Can you work these out from the model? Positions are in its coordinate system, mm. A direction names the side the tool comes from. Give positions to 0.01 mm unless a question says otherwise; leave off trailing zeros. Order: outer loops, then holes, each group sorted by start corner. A loop starts at its lowest first (then second) coordinate and runs counter-clockwise, first axis right, second up. Notation, with made-up numbers: (-7, 40) - (28, 40) arc R12 cw to (28, 53) - close; hole circle Ø11 at (34, 13.5). An arc over 180 degrees is marked (long way). Return JSON: item names as keys, results as strings.
```python
from build123d import *

# Parameters (mm, degrees)
SKETCH1_W           = 21
SKETCH1_H           = 30
SKETCH1_R           = 1.6
BOSS_EXTRUDE3_DEPTH = 10
SKETCH3_W           = 8
SKETCH3_H           = 30
BOSS_EXTRUDE4_DEPTH = 55
SKETCH4_W           = 30
SKETCH4_H           = 10
BOSS_EXTRUDE5_DEPTH = 25
CUT_EXTRUDE1_REACH  = 82.312
SKETCH5_W           = 6.5
SKETCH5_H           = 16.5
SKETCH7_R           = 2.5
CUT_EXTRUDE2_DEPTH  = 17.2
FILLET2_R           = 5
BOSS_EXTRUDE7_START = -10
BOSS_EXTRUDE7_DEPTH = 10


with BuildPart() as part:
    # Sketch1 → Boss-Extrude3 (new body)
    with BuildSketch(Plane(origin=(0, 0, 0), x_dir=(1, 0, 0), z_dir=(0, 1, 0))):
        with Locations((-4.5, -10)):
            Rectangle(SKETCH1_W, SKETCH1_H)
        with Locations(Location((0, 0, 0), (0, 0, 270))):
            Circle(SKETCH1_R, mode=Mode.SUBTRACT)
        with Locations(Location((0, -20, 0), (0, 0, 270))):
            Circle(SKETCH1_R, mode=Mode.SUBTRACT)
    extrude(amount=BOSS_EXTRUDE3_DEPTH)

    # Sketch3 → Boss-Extrude4 (add)
    with BuildSketch(Plane(origin=(0, 10, 0), x_dir=(1, 0, 0), z_dir=(0, 1, 0))):
        with Locations((-11, -10)):
            Rectangle(SKETCH3_W, SKETCH3_H)
    extrude(amount=BOSS_EXTRUDE4_DEPTH)

    # Sketch4 → Boss-Extrude5 (add)
    with BuildSketch(Plane.ZY.offset(15)):
        with Locations((10, 60)):
            Rectangle(SKETCH4_W, SKETCH4_H)
    extrude(amount=BOSS_EXTRUDE5_DEPTH)

    # Sketch5 → Cut-Extrude1 (cut, up to next)
    with BuildSketch(Plane(origin=(0, 65, 0), x_dir=(1, 0, 0), z_dir=(0, 1, 0)), mode=Mode.PRIVATE) as cut_extrude1_sk1:
        with Locations((-31.75, -10)):
            Rectangle(SKETCH5_W, SKETCH5_H)
    cut_extrude1_tool1 = extrude(cut_extrude1_sk1.sketch, amount=-CUT_EXTRUDE1_REACH, mode=Mode.PRIVATE) & part.part
    add(cut_extrude1_tool1.solids().sort_by_distance((-31.75, 65, 10))[0], mode=Mode.SUBTRACT)

    # Sketch7 → Cut-Extrude2 (cut)
    with BuildSketch(Plane.ZY.offset(40)):
        with Locations((10, 60)):
            Circle(SKETCH7_R)
    extrude(amount=-CUT_EXTRUDE2_DEPTH, mode=Mode.SUBTRACT)

    # Fillet2
    fillet2_edges = [part.edges().sort_by_distance(p)[0] for p in [
        (-7, 65, 10),
        (-15, 55, 10),
        (-40, 60, -5),
        (-40, 60, 25),
        (-15, 0, 10),
        (6, 5, -5),
        (6, 5, 25),
    ]]
    fillet(fillet2_edges, radius=FILLET2_R)

    # Sketch8 → Boss-Extrude7 (add)
    with BuildSketch(Plane.XY.offset(25).offset(BOSS_EXTRUDE7_START)):
        Polygon((-7, 10), (-7, 60), (6, 10), align=None)
    extrude(amount=-BOSS_EXTRUDE7_DEPTH)


solid = part.part
```
1. Suppose I cut it at C-C (z = 10). List the corners of the cut face in (x, y) for me, plus the area to 3 significant figures.
Checks:
{"outline": "(-40, 55) - (-35, 55) - (-35, 57.5) - (-40, 57.5) - close; (-40, 62.5) - (-35, 62.5) - (-35, 65) - (-40, 65) - close; (-28.5, 55) - (-20, 55) arc R5 cw to (-15, 50) - (-15, 5) arc R5 ccw to (-10, 0) - (6, 0) - (6, 10) - (-7, 60) arc R5 ccw to (-12, 65) - (-28.5, 65) - (-28.5, 62.5) - (-22.8, 62.5) - (-22.8, 57.5) - (-28.5, 57.5) - close", "area": "1,100 mm^2"}
2. Suppose I cut it at B-B (x = -32.5). List the corners of the cut face in (y, z) for me.
Checks:
{"outline": "(55, -5) - (65, -5) - (65, 1.75) - (55, 1.75) - close; (55, 18.25) - (65, 18.25) - (65, 25) - (55, 25) - close"}
3. For pin 1 Ø3 at (y, z) = (60, 10) entering from +X; pin 2 Ø8 at (x, z) = (-0.5, 22) entering from +Y; pin 3 Ø6.5 at (x, y) = (0.5, 45.5) entering from -Z; pin 4 Ø3 at (y, z) = (24.5, 4) entering from -X, each with a flat end and sliding along its axis, tell me the tip position at first contact or that it passes through.
Checks:
{"pin 1": "x = -6.61", "pin 2": "y = 10", "pin 3": "through", "pin 4": "x = -15"}
4. Suppose I cut it at A-A (z = 6.75). List the corners of the cut face in (x, y) for me, plus the area to 3 significant figures.
Checks:
{"outline": "(-40, 55) - (-35, 55) - (-35, 65) - (-40, 65) - close; (-28.5, 55) - (-20, 55) arc R5 cw to (-15, 50) - (-15, 5) arc R5 ccw to (-10, 0) - (6, 0) - (6, 10) - (-7, 60) arc R5 ccw to (-12, 65) - (-28.5, 65) - close", "area": "1,150 mm^2"}
5. Thinking about a two-plate mould opening in Z: for faces 6 (the face through (-17, 54, 10)), 7 (the face through (-39, 60, 23)), 8 (the face through (-37.53, 57.56, 9.46)), 9 (the face through (-32, 60, 18.25)), which applies, +Z half, -Z half, draft (parallel to the pull), parting line (faces both ways), or undercut?
Checks:
{"face 6": "draft", "face 7": "+Z half", "face 8": "undercut", "face 9": "undercut"}
6. Suppose I cut it at D-D (y = 7). List the corners of the cut face in (x, z) for me, plus the area to 3 significant figures.
Checks:
{"outline": "(-15, -5) - (1, -5) arc R5 ccw to (6, 0) - (6, 20) arc R5 ccw to (1, 25) - (-15, 25) - close; hole circle Ø3.2 at (0, 0); hole circle Ø3.2 at (0, 20)", "area": "603 mm^2"}
7. If I drill on L1, parallel to Y at x = -24.5, z = 10; L2, parallel to Y at x = -27, z = 3.25; L3, parallel to X at y = 34.5, z = -2.75, over which ranges is the centre line in solid material (lowest first)? Write a range as [from, to].
Checks:
{"L1": "[55, 57.5], [62.5, 65]", "L2": "[55, 65]", "L3": "[-15, -7]"}
8. On a 3-axis mill with a long thin cutter (end or side, diameter ignored), from which of +Z, -Z, +X, -X, +Y, -Y can I reach the whole of each face in a straight line? I mean faces 1 (the face through (-15, 27, 10)), 2 (the face through (-25.69, 57.56, 9.46)), 3 (the face through (-7, 35, 0)), 4 (the face through (-28.5, 62, 8)), 5 (the face through (5, 5, 23)). Say none if no direction works.
Checks:
{"face 1": "+Z, -Z, -X, -Y", "face 2": "-X", "face 3": "-Z, +X, +Y", "face 4": "+Y, -Y", "face 5": "+Z, +X, +Y, -Y"}
